Here's how the part is built. I have some questions about the finished solid (model axes, mm). Face numbers are marked on the shaded views. Give positions to 0.01 mm unless a question says otherwise; leave off trailing zeros. Loops run counter-clockwise (first coordinate to the right, second up) from the corner with the lowest first, then second, coordinate; pieces in that order, holes last. Notation, with made-up numbers: (87.25, 78) - (92.25, 78) arc R29 cw to (92.25, 106) - close; hole circle Ø3 at (4, -37). An arc over 180 degrees is marked (long way). Use one line per item in the form item = value.
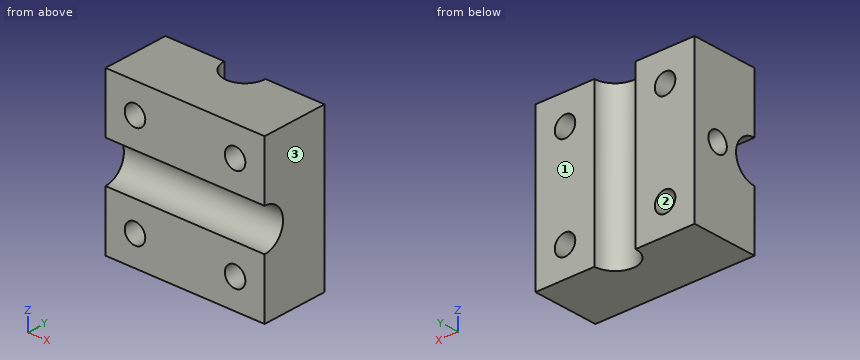
from build123d import *

# Parameters (mm, degrees)
P_IDAT_VYSUNUT_M1_DEPTH  = 31
SKICA2_R                 = 4
ODEBRAT_VYSUNUT_M1_DEPTH = 45.319860108
SKICA3_R                 = 2
ODEBRAT_VYSUNUT_M2_DEPTH = 38.016888038
SKICA4_R                 = 2
ODEBRAT_VYSUNUT_M3_DEPTH = 10


with BuildPart() as part:
    # Skica1 → Přidat vysunutím1 (new body)
    with BuildSketch(Plane.XY):
        with BuildLine():
            Line((-15.5, 6.5), (-4, 6.5))
            ThreePointArc((-4, 6.5), (0, 2.5), (4, 6.5))
            Line((4, 6.5), (15.5, 6.5))
            Line((15.5, 6.5), (15.5, -6.5))
            Line((15.5, -6.5), (-15.5, -6.5))
            Line((-15.5, -6.5), (-15.5, 6.5))
        make_face()
    extrude(amount=P_IDAT_VYSUNUT_M1_DEPTH)

    # Skica2 → Odebrat vysunutím1 (cut, through all)
    with BuildSketch(Plane.ZY.offset(15.5)):
        with Locations((15.5, -6.5)):
            Circle(SKICA2_R)
    extrude(amount=-ODEBRAT_VYSUNUT_M1_DEPTH, mode=Mode.SUBTRACT)

    # Skica3 → Odebrat vysunutím2 (cut, through all)
    with BuildSketch(Plane(origin=(0, 6.5, 0), x_dir=(1, 0, 0), z_dir=(0, 1, 0))):
        with Locations(Location((9.75, -5.75, 0), (0, 0, 270))):
            Circle(SKICA3_R)
        with Locations(Location((9.75, -25.25, 0), (0, 0, 90))):
            Circle(SKICA3_R)
        with Locations(Location((-9.75, -25.25, 0), (0, 0, 270))):
            Circle(SKICA3_R)
        with Locations(Location((-9.75, -5.75, 0), (0, 0, 90))):
            Circle(SKICA3_R)
    extrude(amount=-ODEBRAT_VYSUNUT_M2_DEPTH, mode=Mode.SUBTRACT)

    # Skica4 → Odebrat vysunutím3 (cut)
    with BuildSketch(Plane.ZY.offset(15.5)):
        with Locations((15.5, 1.5)):
            Circle(SKICA4_R)
    extrude(amount=-ODEBRAT_VYSUNUT_M3_DEPTH, mode=Mode.SUBTRACT)


solid = part.part
(1) If we section it at B-B (y = 5): List the corners of the cut face in (x, z) for me, plus the area to 3 significant figures.
Geometry says:
outline = (-15.5, 0) - (-3.71, 0) - (-3.71, 31) - (-15.5, 31) - close; (3.71, 0) - (15.5, 0) - (15.5, 31) - (3.71, 31) - close; hole circle Ø4 at (-9.75, 5.75); hole circle Ø4 at (-9.75, 25.25); hole circle Ø4 at (9.75, 5.75); hole circle Ø4 at (9.75, 25.25)
area = 681 mm²
(2) Thinking about a two-plate mould opening in X: for the marked faces 1, 2 and 3, which applies, pulls with the +X half, pulls with the -X half, needs draft (parallel to the pull), parting line crosses it, or undercut?
Geometry says:
face_1 = needs draft
face_2 = undercut
face_3 = pulls with the +X half
(3) If we section it at D-D (y = -1): List the corners of the cut face in (x, z) for me.
Geometry says:
outline = (-15.5, 0) - (15.5, 0) - (15.5, 31) - (-15.5, 31) - close; hole circle Ø4 at (-9.75, 5.75); hole circle Ø4 at (-9.75, 25.25); hole circle Ø4 at (9.75, 5.75); hole circle Ø4 at (9.75, 25.25)
(4) If we section it at C-C (z = 25.25): List the corners of the cut face in (x, y) for me, plus the area to 3 significant figures.
Geometry says:
outline = (-15.5, -6.5) - (-11.75, -6.5) - (-11.75, 6.5) - (-15.5, 6.5) - close; (-7.75, -6.5) - (7.75, -6.5) - (7.75, 6.5) - (4, 6.5) arc R4 cw to (-4, 6.5) - (-7.75, 6.5) - close; (11.75, -6.5) - (15.5, -6.5) - (15.5, 6.5) - (11.75, 6.5) - close
area = 274 mm²
(5) If we section it at A-A (x = -9.75): List the corners of the cut face in (y, z) for me.
Geometry says:
outline = (-6.5, 0) - (6.5, 0) - (6.5, 3.75) - (-6.5, 3.75) - close; (-6.5, 7.75) - (6.5, 7.75) - (6.5, 23.25) - (-6.5, 23.25) - (-6.5, 19.5) arc R4 cw to (-6.5, 11.5) - close; (-6.5, 27.25) - (6.5, 27.25) - (6.5, 31) - (-6.5, 31) - close; hole circle Ø4 at (1.5, 15.5)
(6) If I drill on probe 1 along X at (y, z) = (-2.5, 5.75); probe 2 along Y at (x, z) = (-12.25, 15.5); probe 3 along Z at (x, y) = (-11.5, 4), over which ranges is the centre line in solid material (lowest first)?
Geometry says:
probe_1 = -15.5 to -11.75, -7.75 to 7.75, 11.75 to 15.5
probe_2 = -2.5 to -0.5, 3.5 to 6.5
probe_3 = 0 to 4.78, 6.72 to 24.28, 26.22 to 31
(7) For P1, Ø3, axis at x = -9.75, z = 5.75, coming from the -Y side; P2, Ø1, axis at y = 1.5, z = 15.5, coming from the -X side, each with a flat end and sliding along its axis, tell me the tip position at first contact or that it passes through.
Geometry says:
P1 = through
P2 = -5.5
